from build123d import *

# Parameters (mm, degrees)
F1_DEPTH = 5.3


with BuildPart() as f1:
    # F0 (on Top) → F1 (new body)
    with BuildSketch(Plane.XY):
        with BuildLine():
            ThreePointArc((-5.026474, 3.543595), (-1.858721, -5.862393), (6.15, 0))
            ThreePointArc((6.15, 0), (5.859092, 1.869103), (5.013888, 3.56138))
            Line((5.013888, 3.56138), (3.013888, 3.56138))
            Line((3.013888, 3.56138), (1.287191, 1.095401))
            Line((1.287191, 1.095401), (1.55, 0.91138))
            Line((1.55, 0.91138), (3.85, 0.91138))
            Line((3.85, 0.91138), (3.85, -1.38862))
            Line((3.85, -1.38862), (1.55, -1.38862))
            Line((1.55, -1.38862), (1.15, -1.55))
            Line((1.15, -1.55), (1.15, -3.85))
            Line((1.15, -3.85), (-1.15, -3.85))
            Line((-1.15, -3.85), (-1.15, -1.55))
            Line((-1.15, -1.55), (-1.55, -1.406405))
            Line((-1.55, -1.406405), (-3.85, -1.406405))
            Line((-3.85, -1.406405), (-3.85, 0.893595))
            Line((-3.85, 0.893595), (-1.55, 0.893595))
            Line((-1.55, 0.893595), (-1.328561, 1.118723))
            Line((-1.328561, 1.118723), (-3.026474, 3.543595))
            Line((-3.026474, 3.543595), (-5.026474, 3.543595))
        make_face()
    extrude(amount=F1_DEPTH)


solid = f1.part
Source: CAD feature listing. Evaluate the final solid. Frame: model axes, mm. A direction names the side the tool comes from. Coordinates: 2 decimals unless noted, no trailing zeros. Loops run counter-clockwise (first coordinate to the right, second up) from the corner with the lowest first, then second, coordinate; pieces in that order, holes last. Notation, with made-up numbers: (26, 56) - (53, 56) arc R31 cw to (53, 87) - close; hole circle Ø11 at (3.5, 70.5). An arc over 180 degrees is marked (long way). Return JSON: item names as keys, results as strings.
Q1. Section B-B, the plane y = -3. Return loops of the section in (x, z), plus the area to 3 significant figures.
Results:
{"outline": "(-5.37, 0) - (-1.15, 0) - (-1.15, 5.3) - (-5.37, 5.3) - close; (1.15, 0) - (5.37, 0) - (5.37, 5.3) - (1.15, 5.3) - close", "area": "44.7 mm2"}
Q2. Section A-A, the plane z = 3.25. Return loops of the section in (x, y), plus the area to 3 significant figures.
Results:
{"outline": "(-5.03, 3.54) arc R6.15 ccw (long way) to (6.15, 0) arc R6.15 ccw to (5.01, 3.56) - (3.01, 3.56) - (1.29, 1.1) - (1.55, 0.91) - (3.85, 0.91) - (3.85, -1.39) - (1.55, -1.39) - (1.15, -1.55) - (1.15, -3.85) - (-1.15, -3.85) - (-1.15, -1.55) - (-1.55, -1.41) - (-3.85, -1.41) - (-3.85, 0.89) - (-1.55, 0.89) - (-1.33, 1.12) - (-3.03, 3.54) - close", "area": "66.0 mm2"}
Q3. Contact query for flat-ended pins moving along their axis: P1, Ø1.2, axis at x = -3, z = 3.5, coming from the +Y side; P2, Ø2.5, axis at x = 0.5, z = 1.5, coming from the +Y side; P3, Ø0.7, axis at y = -0.5, z = 3.5, coming from the +X side; P4, Ø2, axis at x = 3.5, y = -3, coming from the -Z side. Output: stop coordinate, or through.
Results:
{"P1": "y = 3.54", "P2": "y = 1.76", "P3": "x = 6.15", "P4": "z = 0"}
Q4. Material intervals for line 1 along X through (y, z) = (0.25, 1.2); line 2 along Y through (x, z) = (-3, 4.75); line 3 along X through (y, z) = (3.25, 4.75), sorted ascending.
Results:
{"line 1": "-6.14 to -3.85, 3.85 to 6.14", "line 2": "-5.37 to -1.41, 0.89 to 3.51", "line 3": "-5.22 to -2.82, 2.8 to 5.22"}
Q5. Mould query, pull axis Y, two halves, no side actions, for faces 4 (the flat face through (-3.85, 0, 3)), 5 (the flat face through (-1.5, -2.3, 5.3)), 6 (the flat face through (-4, 3.544, 3)). Classes: released by +Y, released by -Y, zero draft, split by the parting line, or undercut.
Results:
{"face 4": "undercut", "face 5": "zero draft", "face 6": "released by +Y"}
Q6. Access query for faces 1 (the flat face through (-3, 0.894, 3)), 2 (the flat face through (4, 3.561, 3)), 3 (the flat face through (2.163, 2.346, 2.613)). Directions: +Z, -Z, +X, -X, +Y, -Y. A direction counts if a zero-diameter tool reaches every point of the face in a straight line with its end or side. Return the directions, or none.
Results:
{"face 1": "+Z, -Z", "face 2": "+Z, -Z, +X, -X, +Y", "face 3": "+Z, -Z, +Y"}
Q7. Section C-C, the plane x = -2.75. Return loops of the section in (y, z), plus the area to 3 significant figures.
Results:
{"outline": "(-5.5, 0) - (-1.41, 0) - (-1.41, 5.3) - (-5.5, 5.3) - close; (0.89, 0) - (3.15, 0) - (3.15, 5.3) - (0.89, 5.3) - close", "area": "33.7 mm2"}
Q8. Section D-D, the plane x = 0. Return loops of the section in (y, z).
Results:
{"outline": "(-6.15, 0) - (-3.85, 0) - (-3.85, 5.3) - (-6.15, 5.3) - close"}
